from build123d import *

# Parameters (mm, degrees)
SKETCH1_W                          = 10
SKETCH1_H                          = 30
BASE_FLANGE1_DEPTH                 = 1.75
EDGE_FLANGE1_DEPTH                 = 30
M3_CLEARANCE_HOLE1_D               = 3.4
M3_CLEARANCE_HOLE1_DEPTH           = 5
M3_CLEARANCE_HOLE1_TIP             = 1.021463052
M3_CLEARANCE_HOLE1_ON_FACE_2_D     = 3.4
M3_CLEARANCE_HOLE1_ON_FACE_2_DEPTH = 5
M3_CLEARANCE_HOLE1_ON_FACE_2_TIP   = 1.021463052


# Sheet-metal steps are written as plain solids
with BuildPart() as part:
    # Sketch1 → Base-Flange1 (new body)
    with BuildSketch(Plane.XY):
        with Locations((5, 15)):
            Rectangle(SKETCH1_W, SKETCH1_H)
    extrude(amount=-BASE_FLANGE1_DEPTH)

    # Edge-Flange1 section (across the edge) → Edge-Flange1 (add)
    with BuildSketch(Plane(origin=(-1.75, 30, 0), x_dir=(1, 0, 0), z_dir=(0, -1, 0))):
        with BuildLine():
            Line((-1.75, 1.75), (-1.75, 11.25))
            Line((-1.75, 11.25), (0, 11.25))
            Line((0, 11.25), (0, 1.75))
            ThreePointArc((0, 1.75), (0.512563133, 0.512563133), (1.75, 0))
            Line((1.75, 0), (1.75, -1.75))
            ThreePointArc((1.75, -1.75), (-0.724873734, -0.724873734), (-1.75, 1.75))
        make_face()
    extrude(amount=EDGE_FLANGE1_DEPTH)

    # M3 Clearance Hole1
    with Locations(Plane(origin=(5, 22, 0), x_dir=(1, 0, 0), z_dir=(0, 0, 1))):
        with Locations((0, 0), (0, -14)):
            Hole(M3_CLEARANCE_HOLE1_D / 2, depth=M3_CLEARANCE_HOLE1_DEPTH)
            with Locations((0, 0, -(M3_CLEARANCE_HOLE1_DEPTH + M3_CLEARANCE_HOLE1_TIP / 2))):  # 118° drill point
                Cone(0, M3_CLEARANCE_HOLE1_D / 2, M3_CLEARANCE_HOLE1_TIP, mode=Mode.SUBTRACT)

    # M3 Clearance Hole1 on face 2
    with Locations(Plane(origin=(-1.75, 22, 6.5), x_dir=(0, 0, 1), z_dir=(1, 0, 0))):
        with Locations((0, 0), (0, 14)):
            Hole(M3_CLEARANCE_HOLE1_ON_FACE_2_D / 2, depth=M3_CLEARANCE_HOLE1_ON_FACE_2_DEPTH)
            with Locations((0, 0, -(M3_CLEARANCE_HOLE1_ON_FACE_2_DEPTH + M3_CLEARANCE_HOLE1_ON_FACE_2_TIP / 2))):  # 118° drill point
                Cone(0, M3_CLEARANCE_HOLE1_ON_FACE_2_D / 2, M3_CLEARANCE_HOLE1_ON_FACE_2_TIP, mode=Mode.SUBTRACT)


solid = part.part
Input: part model. Units: mm. Frame: model coordinates. A direction names the side the tool comes from. Coordinates: 2 decimals unless noted, no trailing zeros. Loops run counter-clockwise (first coordinate to the right, second up) from the corner with the lowest first, then second, coordinate; pieces in that order, holes last.
(1) First-contact query: pin 1 Ø2 at (y, z) = (23.5, 5.5) entering from +X; pin 2 Ø4 at (x, y) = (5, 22) entering from +Z; pin 3 Ø4 at (x, y) = (0.5, 21) entering from +Z. Flat tips, straight axial feed; report the tip coordinate or a pass-through.
(2) Set-up query: faces 5 (the face through (5, 15, 0)), 6 (the face through (5.221, 23.686, -0.887)). Return all of +Z, -Z, +X, -X, +Y, -Y with unobstructed straight access to the full face (end or side cutting, diameter ignored); none if empty.
(3) Section C-C on y = 8. Return the cut outline in (x, z), then the cut area to 3 significant figures.
(4) Pull-direction query (Z, two-part tool) for faces 1 (the face through (-2.637, 20.314, 6.721)), 2 (the face through (-2.4, 15.2, -0.8)), 3 (the face through (-2.64, 9.66, 6.87)), 4 (the face through (-1.75, 15, 7)); classes: released by +Z, released by -Z, zero draft, split by the parting line, or undercut.
(5) Section A-A on z = 6.5. Return the cut outline in (x, y).
(6) Section B-B on x = 5. Return the cut outline in (y, z).
(7) Material intervals for probe 1 along Y at (x, z) = (-2.05, 6.5); probe 2 along Z at (x, y) = (6.75, 9.75); probe 3 along X at (y, z) = (26.25, 4.5), sorted ascending.
(8) Section D-D on y = 13.75. Return the cut outline in (x, z).
Data:
1. pin 1: stops at x = -1.75
1. pin 2: stops at z = 0
1. pin 3: stops at z = 0.85
2. face 5: +Z, +X, +Y, -Y
2. face 6: +Z, -Z
3. outline: (-3.5, 1.75) arc R3.5 ccw to (0, -1.75) - (3.3, -1.75) - (3.3, 0) - (0, 0) arc R1.75 cw to (-1.75, 1.75) - (-1.75, 4.8) - (-3.5, 4.8) - close; (-3.5, 8.2) - (-1.75, 8.2) - (-1.75, 11.25) - (-3.5, 11.25) - close; (6.7, -1.75) - (10, -1.75) - (10, 0) - (6.7, 0) - close
3. area: 29.4 mm2
4. face 1: undercut
4. face 2: released by -Z
4. face 3: undercut
4. face 4: zero draft
5. outline: (-3.5, 0) - (-1.75, 0) - (-1.75, 6.3) - (-3.5, 6.3) - close; (-3.5, 9.7) - (-1.75, 9.7) - (-1.75, 20.3) - (-3.5, 20.3) - close; (-3.5, 23.7) - (-1.75, 23.7) - (-1.75, 30) - (-3.5, 30) - close
6. outline: (0, -1.75) - (6.3, -1.75) - (6.3, 0) - (0, 0) - close; (9.7, -1.75) - (20.3, -1.75) - (20.3, 0) - (9.7, 0) - close; (23.7, -1.75) - (30, -1.75) - (30, 0) - (23.7, 0) - close
7. probe 1: y = 0 to 6.3, 9.7 to 20.3, 23.7 to 30
7. probe 2: z = -1.75 to 0
7. probe 3: x = -3.5 to -1.75
8. outline: (-3.5, 1.75) arc R3.5 ccw to (0, -1.75) - (10, -1.75) - (10, 0) - (0, 0) arc R1.75 cw to (-1.75, 1.75) - (-1.75, 11.25) - (-3.5, 11.25) - close
